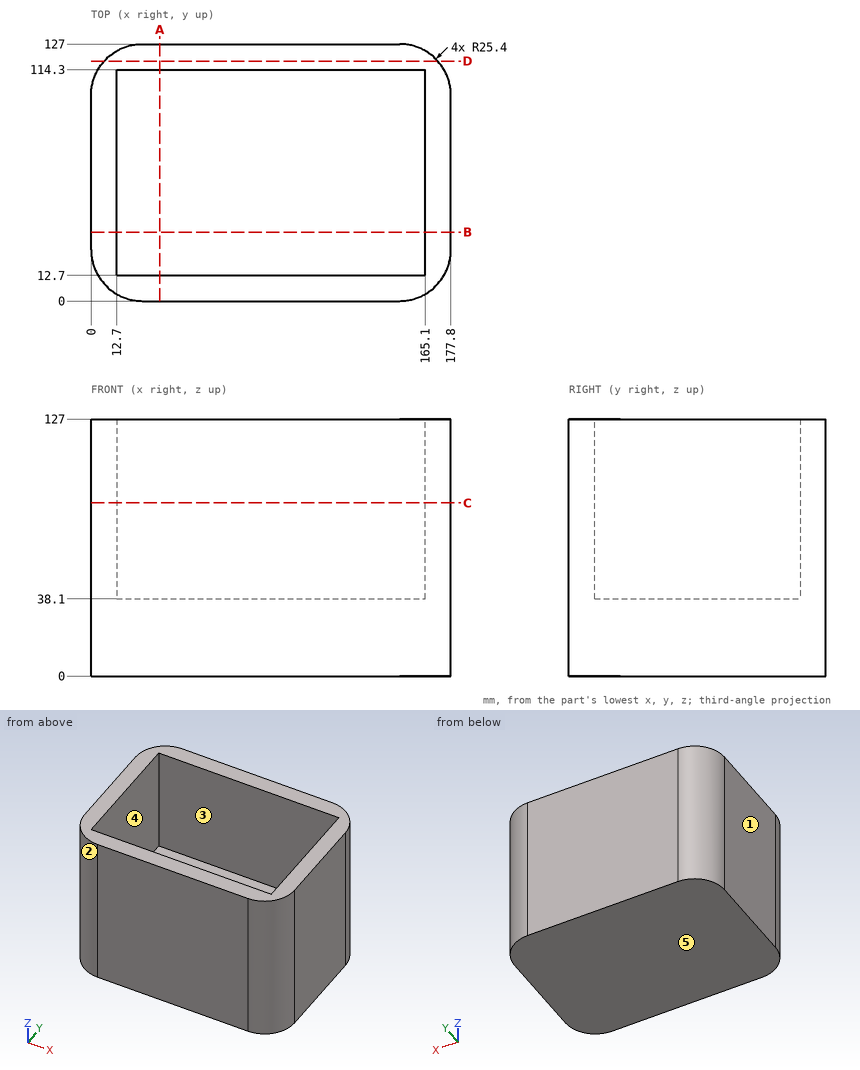
Verification items for this drawing (mm, ordinates from the low corner). A direction names the side the tool comes from. Coordinates: 2 decimals unless noted, no trailing zeros. Loops run counter-clockwise (first coordinate to the right, second up) from the corner with the lowest first, then second, coordinate; pieces in that order, holes last. Notation, with made-up numbers: (38.5, -20.75) -> (95.5, -20.75) arc R18 cw to (95.5, -8.75) -> close; hole circle Ø2 at (7, 69). An arc over 180 degrees is marked (long way). Answer in a Markdown table with one row per item. Add a question column.
1. Section check D-D, the plane y = 118.5. Enter the section's corners in (x, z).
2. Draft check along Y on the marked faces 1, 2 and 3. Enter one of: +Y half, -Y half, draft (parallel to the pull), parting line (faces both ways), or undercut.
3. Material ranges on probe 1 along X at (y, z) = (31, 111); probe 2 along Y at (x, z) = (84.5, 92); probe 3 along Z at (x, y) = (40, 67.5), recorded low to high. Write a range as [from, to].
4. Access from +Z, -Z, +X, -X, +Y, -Y to the whole of each face (thin tool, end or side, straight path). Record for the marked faces 4 and 5.
5. Section check B-B, the plane y = 34. Enter the section's corners in (x, z), then the cut area to 3 significant figures.
6. Section check A-A, the plane x = 34. Enter the section's corners in (y, z).
7. Depth check by flat-ended pin: P1, Ø2, axis at y = 107.5, z = 82, coming from the -X side; P2, Ø5, axis at y = 15.5, z = 76.5, coming from the +X side. Enter the tip coordinate at first touch or a pass-through.
8. Section check C-C, the plane z = 85.5. Enter the section's corners in (x, y), then the cut area to 3 significant figures.
Derived:
| question | item | result |
|---|---|---|
| 1 | outline | (6.44, 0) -> (171.36, 0) -> (171.36, 127) -> (6.44, 127) -> close |
| 2 | face 1 | draft |
| 2 | face 2 | -Y half |
| 2 | face 3 | undercut |
| 3 | probe 1 | x = [0, 12.7], [165.1, 177.8] |
| 3 | probe 2 | y = [0, 12.7], [114.3, 127] |
| 3 | probe 3 | z = [0, 38.1] |
| 4 | face 4 | +Z |
| 4 | face 5 | -Z, +X, -X, +Y, -Y |
| 5 | outline | (0, 0) -> (177.8, 0) -> (177.8, 127) -> (165.1, 127) -> (165.1, 38.1) -> (12.7, 38.1) -> (12.7, 127) -> (0, 127) -> close |
| 5 | area | 9,030 mm² |
| 6 | outline | (0, 0) -> (127, 0) -> (127, 127) -> (114.3, 127) -> (114.3, 38.1) -> (12.7, 38.1) -> (12.7, 127) -> (0, 127) -> close |
| 7 | P1 | stops at x = 0.48 |
| 7 | P2 | stops at x = 176.7 |
| 8 | outline | (0, 25.4) arc R25.4 ccw to (25.4, 0) -> (152.4, 0) arc R25.4 ccw to (177.8, 25.4) -> (177.8, 101.6) arc R25.4 ccw to (152.4, 127) -> (25.4, 127) arc R25.4 ccw to (0, 101.6) -> close; hole (12.7, 12.7) -> (165.1, 12.7) -> (165.1, 114.3) -> (12.7, 114.3) -> close |
| 8 | area | 6,540 mm² |
